```python
from build123d import *

# Parameters (mm, degrees)
BOSS_EXTRUDE1_DEPTH = 0.3175
FILLET1_R           = 0.508


with BuildPart() as part:
    # Sketch2 → Boss-Extrude1 (new body, symmetric)
    with BuildSketch(Plane(origin=(0, 0, 0), x_dir=(1, 0, 0), z_dir=(0, 1, 0))):
        with BuildLine():
            Line((-3.175, 0), (-2.286, 0))
            ThreePointArc((-2.286, 0), (-2.086822944, -0.933255592), (-1.524, -1.703883799))
            Line((-1.524, -1.703883799), (-1.905, -4.434100924))
            ThreePointArc((-1.905, -4.434100924), (0, 4.826), (1.905, -4.434100924))
            Line((1.905, -4.434100924), (1.524, -1.703883799))
            ThreePointArc((1.524, -1.703883799), (2.086822944, -0.933255592), (2.286, 0))
            Line((2.286, 0), (3.175, 0))
            ThreePointArc((3.175, 0), (2.4999975, 1.957201446), (0.762, 3.082203919))
            Line((0.762, 3.082203919), (0.54864, 2.219186822))
            ThreePointArc((0.54864, 2.219186822), (0, 2.286), (-0.54864, 2.219186822))
            Line((-0.54864, 2.219186822), (-0.762, 3.082203919))
            ThreePointArc((-0.762, 3.082203919), (-2.4999975, 1.957201446), (-3.175, 0))
        make_face()
    extrude(amount=BOSS_EXTRUDE1_DEPTH, both=True)

    # Fillet1
    fillet1_edges = [part.edges().sort_by_distance(p)[0] for p in [
        (-1.905, 0, 4.434100924),
        (1.905, 0, 4.434100924),
    ]]
    fillet(fillet1_edges, radius=FILLET1_R)


solid = part.part
```
Build history of the part. All positions in model axes, mm. A direction names the side the tool comes from. Round coordinates to 2 decimals unless told otherwise and drop trailing zeros. Loops run counter-clockwise (first coordinate to the right, second up) from the corner with the lowest first, then second, coordinate; pieces in that order, holes last.
Item 1: Which spindle directions (+Z, -Z, +X, -X, +Y, -Y) get a long thin tool onto all of the face, cutting with end or side? Do faces 4 (the face through (-2.48, 0, -1.98)), 5 (the face through (0, 0.318, -3)). Say none if no direction does.
Item 2: Saw through at D-D (z = -2.75). List the corners of the cut face in (x, y), then the cut area to 3 significant figures.
Item 3: Drill centre lines: line 1 along X through (y, z) = (0.2, -2.5); line 2 along Z through (x, y) = (2.5, -0.15); line 3 along X through (y, z) = (-0.1, 3). Where is each one in solid material? Low to high.
Item 4: Saw through at A-A (z = 2.5). List the corners of the cut face in (x, y), then the cut area to 3 significant figures.
Item 5: Saw through at B-B (y = -0.15). List the corners of the cut face in (x, z) (3 decimals).
Item 6: Two-plate mould, pull along X, no slides. Class faces 1 (the face through (-0.174, 0.004, -4.823)), 2 (the face through (0, -0.318, -3)), 3 (the face through (2.52, 0, -1.93)): released by +X, released by -X, zero draft, split by the parting line, or undercut.
Item 7: Pin check, flat tip, straight feed: P1, Ø1, axis at x = 0.5, z = 3, coming from the -Y side. Stop position of the tip, or through.
Item 8: Saw through at C-C (x = 2). List the corners of the cut face in (y, z).
Worked answers:
1. face 4: +Y, -Y
1. face 5: +Z, -Z, +X, -X, +Y
2. outline: (-3.97, -0.32) - (-1.59, -0.32) - (-1.59, 0.32) - (-3.97, 0.32) - close; (-0.68, -0.32) - (0.68, -0.32) - (0.68, 0.32) - (-0.68, 0.32) - close; (1.59, -0.32) - (3.97, -0.32) - (3.97, 0.32) - (1.59, 0.32) - close
2. area: 3.88 mm2
3. line 1: x = -4.13 to -1.96, -0.62 to 0.62, 1.96 to 4.13
3. line 2: z = -4.13 to -1.96, 0 to 4.12
3. line 3: x = -3.78 to -1.7, 1.7 to 3.78
4. outline: (-4.13, -0.32) - (-1.64, -0.32) - (-1.64, 0.32) - (-4.13, 0.32) - close; (1.64, -0.32) - (4.13, -0.32) - (4.13, 0.32) - (1.64, 0.32) - close
4. area: 3.17 mm2
5. outline: (-3.175, 0) - (-2.286, 0) arc R2.286 cw to (-1.524, 1.704) - (-1.805, 3.719) arc R0.508 ccw to (-2.58, 4.078) arc R4.826 ccw (long way) to (2.58, 4.078) arc R0.508 ccw to (1.805, 3.719) - (1.524, 1.704) arc R2.286 cw to (2.286, 0) - (3.175, 0) arc R3.175 cw to (0.762, -3.082) - (0.549, -2.219) arc R2.286 cw to (-0.549, -2.219) - (-0.762, -3.082) arc R3.175 cw to start
6. face 1: split by the parting line
6. face 2: zero draft
6. face 3: undercut
7. P1: passes through
8. outline: (-0.32, -4.39) - (0.32, -4.39) - (0.32, -2.47) - (-0.32, -2.47) - close; (-0.32, 1.11) - (0.32, 1.11) - (0.32, 4.05) - (-0.32, 4.05) - close
